Part model, mm, in its own coordinate system. Round coordinates to 2 decimals unless told otherwise and drop trailing zeros. Write each loop counter-clockwise with the first axis right and the second up, starting at its lowest first coordinate (ties: lowest second). Pieces come first, ordered by that corner, then holes. Notation, with made-up numbers: M 66,54.25 L 112,54.25 A32 cw 112,89.25 Z; hole C 74,72 d1. An arc over 180 degrees is marked long. One line per question, with ' | ' between items. Start each with the question number.
1) Saw through at C-C (z = 1.25). Give the number of separate pieces and of enclosed holes in the cut face, plus the area to 3 significant figures.
2) Saw through at B-B (y = 50). List the corners of the cut face in (x, z).
3) Saw through at A-A (x = 30). List the corners of the cut face in (y, z).
4) Drop a flat-ended pin along its axis: pin 1 Ø12 at (x, y) = (31, 13.5) entering from -Z. Give the stop position or say it passes through.
5) Wall check: probe 1 along Y at (x, z) = (10, 1); probe 2 along Y at (x, z) = (70, 1); probe 3 along X at (y, z) = (12, 1.3). Give the ranges that are in metal, low to high. Write a range as [from, to].
```python
from build123d import *

# Parameters (mm, degrees)
EXTRUDE_1_DEPTH       = 2
HOLE_WIZARD_M41_D     = 4.5
HOLE_WIZARD_M41_DEPTH = 5
HOLE_WIZARD_M41_TIP   = 1.351936393


with BuildPart() as part:
    # Эскиз1 → Бобышка-Вытянуть1 (new body)
    with BuildSketch(Plane.XY):
        Polygon((0, 0), (0, 80), (40, 80), (80, 40), (80, 0), align=None)
    extrude(amount=EXTRUDE_1_DEPTH)

    # Отверстие с зазором M41
    with Locations(Plane(origin=(0, 0, 0), x_dir=(-1, 0, 0), z_dir=(0, 0, -1))):
        with Locations((-70, 10), (-30, 50), (-50, 10), (-10, 50), (-70, 30), (-30, 70), (-50, 30), (-10, 70), (-30, 10), (-10, 10), (-30, 30), (-10, 30)):
            Hole(HOLE_WIZARD_M41_D / 2, depth=HOLE_WIZARD_M41_DEPTH)
            with Locations((0, 0, -(HOLE_WIZARD_M41_DEPTH + HOLE_WIZARD_M41_TIP / 2))):  # 118° drill point
                Cone(0, HOLE_WIZARD_M41_D / 2, HOLE_WIZARD_M41_TIP, mode=Mode.SUBTRACT)


solid = part.part
```
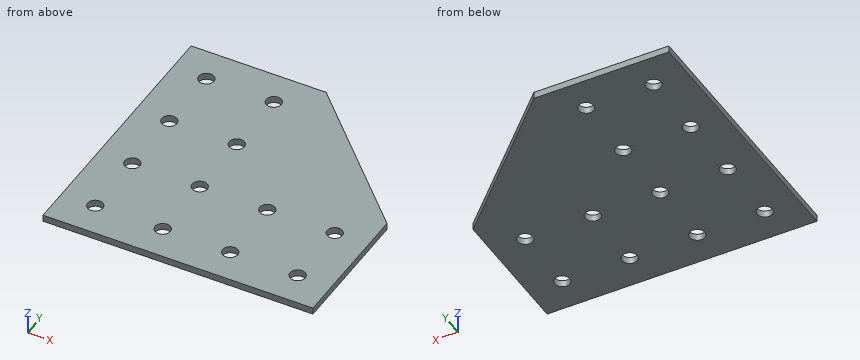
Answer key:
1) separate pieces: 1 | enclosed holes: 12 | area: 5,410 mm2
2) outline: M 0,0 L 7.75,0 L 7.75,2 L 0,2 Z; M 12.25,0 L 27.75,0 L 27.75,2 L 12.25,2 Z; M 32.25,0 L 70,0 L 70,2 L 32.25,2 Z
3) outline: M 0,0 L 7.75,0 L 7.75,2 L 0,2 Z; M 12.25,0 L 27.75,0 L 27.75,2 L 12.25,2 Z; M 32.25,0 L 47.75,0 L 47.75,2 L 32.25,2 Z; M 52.25,0 L 67.75,0 L 67.75,2 L 52.25,2 Z; M 72.25,0 L 80,0 L 80,2 L 72.25,2 Z
4) pin 1: stops at z = 0
5) probe 1: y = [0, 7.75], [12.25, 27.75], [32.25, 47.75], [52.25, 67.75], [72.25, 80] | probe 2: y = [0, 7.75], [12.25, 27.75], [32.25, 50] | probe 3: x = [0, 8.97], [11.03, 28.97], [31.03, 48.97], [51.03, 68.97], [71.03, 80]
